Could you check a few things on this model? Use its own coordinates, in mm. A direction names the side the tool comes from. Give positions to 0.01 mm unless a question says otherwise; leave off trailing zeros. Loops run counter-clockwise (first coordinate to the right, second up) from the corner with the lowest first, then second, coordinate; pieces in that order, holes last. Notation, with made-up numbers: M -14,12.5 L 24,12.5 A23 ccw 24,50.5 Z; hole C 76.25,-29 d7. An arc over 180 degrees is marked long. Return JSON: item names as keys, results as strings. Group by question number.
1. If we section it at B-B (y = 19): Write out the boundary of the cut face in (x, z), plus the area to 3 significant figures.
2. If we mould it in two halves opening along Z, with no side actions, what happens to faces 1 (the flat face through (-8, 24, 9)), 2 (the flat face through (2.3, 2, 1.2)), 3 (the flat face through (-10, 24, -8))? For each: +Z half, -Z half, draft (parallel to the pull), parting line (faces both ways), or undercut.
3. If we section it at C-C (z = -19): Write out the boundary of the cut face in (x, y), plus the area to 3 significant figures.
4. If we section it at A-A (z = 0): Write out the boundary of the cut face in (x, y).
5. If we section it at D-D (z = -8.5): Write out the boundary of the cut face in (x, y).
6. Please list where these lines run through material, in increasing order: line 1 (X direction, y = 0.55, z = 0); line 2 (X direction, y = 32, z = -20.5); line 3 (Y direction, x = -2.5, z = -4).
7. For faces 4 (the cylindrical face through (24.844, 24.336, 6.947)), 5 (the cylindrical face through (-4.88, 0.99, 1.08)), 6 (the flat face through (17, 24, -10)), which set-ups out of +Z, -Z, +X, -X, +Y, -Y let a thin tool reach every point of the face, with its end or its side?
8. For pin 1 (6 mm diameter, centred on y = 31.5, z = -18.5, fed in from +X); pin 2 (8 mm diameter, centred on x = 0, z = 0, fed in from -Y); pin 3 (6 mm diameter, centred on x = 17, y = 30.5, fed in from -Z), each with a flat end and sliding along its axis, tell me the tip position at first contact or that it passes through.
```python
from build123d import *

# Parameters (mm, degrees)
BOSS_EXTRUDE1_DEPTH  = 48
M4_CLEARANCE_HOLE1_D = 4.8
SKETCH4_R            = 5
CUT_EXTRUDE1_DEPTH   = 2
CHAMFER1_SIZE        = 3
FILLET1_R            = 2


with BuildPart() as part:
    # Sketch1 → Boss-Extrude1 (new body)
    with BuildSketch(Plane(origin=(0, 0, 0), x_dir=(1, 0, 0), z_dir=(0, 1, 0))):
        Polygon((-10, 10), (-10, 25), (10, 25), (10, 10), (25, 10), (25, -10), (10, -10), (-10, -10), align=None)
    extrude(amount=BOSS_EXTRUDE1_DEPTH)

    # M4 Clearance Hole1 (through all)
    with Locations(Plane(origin=(0, 48, 0), x_dir=(1, 0, 0), z_dir=(0, 1, 0))):
        with Locations((0, 0)):
            Hole(M4_CLEARANCE_HOLE1_D / 2)

    # Sketch4 → Cut-Extrude1 (cut)
    with BuildSketch(Plane.XZ):
        with Locations(Location((0, 0, 0), (0, 0, 270))):
            Circle(SKETCH4_R)
    extrude(amount=-CUT_EXTRUDE1_DEPTH, mode=Mode.SUBTRACT)

    # Chamfer1
    chamfer1_edges = [part.edges().sort_by_distance(p)[0] for p in [
        (-10, 24, -25),
        (10, 24, -25),
        (10, 24, -10),
        (25, 24, -10),
        (25, 24, 10),
        (-10, 24, 10),
    ]]
    chamfer(chamfer1_edges, length=CHAMFER1_SIZE)

    # Fillet1
    fillet1_edges = [part.edges().sort_by_distance(p)[0] for p in [
        (10, 24, -22),
        (10, 24, -13),
        (22, 24, -10),
        (13, 24, -10),
        (-10, 24, 7),
        (-10, 24, -22),
        (7, 24, -25),
        (-7, 24, -25),
        (25, 24, 7),
        (25, 24, -7),
        (-7, 24, 10),
        (22, 24, 10),
    ]]
    fillet(fillet1_edges, radius=FILLET1_R)


solid = part.part
```
Answer:
{
 "1": {"outline": "M -10,-21.17 A2 ccw -9.41,-22.59 L -7.59,-24.41 A2 ccw -6.17,-25 L 6.17,-25 A2 ccw 7.59,-24.41 L 9.41,-22.59 A2 ccw 10,-21.17 L 10,-13.83 A2 cw 10.59,-12.41 L 12.41,-10.59 A2 cw 13.83,-10 L 21.17,-10 A2 ccw 22.59,-9.41 L 24.41,-7.59 A2 ccw 25,-6.17 L 25,6.17 A2 ccw 24.41,7.59 L 22.59,9.41 A2 ccw 21.17,10 L -6.17,10 A2 ccw -7.59,9.41 L -9.41,7.59 A2 ccw -10,6.17 Z; hole C 0,0 d4.8", "area": "963 mm²"},
 "2": {"face 1": "+Z half", "face 2": "undercut", "face 3": "draft"},
 "3": {"outline": "M -10,0 L 10,0 L 10,48 L -10,48 Z", "area": "960 mm²"},
 "4": {"outline": "M -10,0 L -5,0 L -5,2 L -2.4,2 L -2.4,48 L -10,48 Z; M 2.4,2 L 5,2 L 5,0 L 25,0 L 25,48 L 2.4,48 Z"},
 "5": {"outline": "M -10,0 L 23.5,0 L 23.5,48 L -10,48 Z"},
 "6": {"line 1": "x = -10 to -5, 5 to 25", "line 2": "x = -10 to 10", "line 3": "y = 2 to 48"},
 "7": {"face 4": "+Z, +X, +Y, -Y", "face 5": "-Y", "face 6": "-Z, +X, +Y, -Y"},
 "8": {"pin 1": "stops at x = 10", "pin 2": "stops at y = 2", "pin 3": "stops at z = -10"}
}
